Autodesk Inventor part; units mm, degrees
ref_plane "YZ Plane" through (0, 0, 0) normal (1, 0, 0) x (0, 1, 0)
ref_plane "XZ Plane" through (0, 0, 0) normal (0, 1, 0) x (-1, 0, 0)
ref_plane "XY Plane" through (0, 0, 0) normal (0, 0, 1) x (1, 0, 0)
sketch "Sketch9" plane through (0, 0, 0) normal (0, 1, 0) x (-1, 0, 0)
  line L0 (25, 25) -> (-25, 25)
  line L1 (-25, 25) -> (-25, -25)
  line L2 (-25, -25) -> (25, -25)
  line L3 (25, -25) -> (25, 25)
  line L4 (25, 25) -> (-25, -25) construction
  line L5 (-25, 25) -> (25, -25) construction
  line L6 (-23, 23) -> (23, 23)
  line L7 (23, 23) -> (23, -23)
  line L8 (23, -23) -> (-23, -23)
  line L9 (-23, -23) -> (-23, 23)
  point P0 (0, 0)
  dimension "d172" = 50
  dimension "d173" = 50
  dimension "d174" = 2
extrude "Extrusion3" add sketch "Sketch9" against normal blind 1180
sketch "Sketch10" plane through (0, 0, 0) normal (1, 0, 0) x (0, 1, 0)
  line L0 (0, 25) -> (0, -25) construction
  line L1 (0, 25) -> (-1180, 25) construction
  line L2 (-1180, -25) -> (-1180, 25) construction
  line L3 (0, -25) -> (-1180, -25) construction
  line L4 (-1175, 8.5) -> (-1158, 8.5)
  line L5 (-1158, 8.5) -> (-1158, -8.5)
  line L6 (-1158, -8.5) -> (-1175, -8.5)
  line L7 (-1175, -8.5) -> (-1175, 8.5)
  line L8 (-1175, 8.5) -> (-1158, -8.5) construction
  line L9 (-1158, 8.5) -> (-1175, -8.5) construction
  circle A0 centre (-1166.5, 0) radius 8.5
  line L10 (0, 25) -> (0, -25)
  point P0 (0, 0)
  point P1 (0, 0)
  point P2 (-1180, 0)
  dimension "d177" = 17
  dimension "d178" = 17
  dimension "d191" = 5
extrude "Extrusion4" cut sketch "Sketch10" along normal through all contours A0
pattern_linear "Rectangular Pattern4" count 10 spacing 125 along (0, 1, 0) of "Extrusion4"
properties part number "TKS 3533 FDS WAY tube3" material "Stainless Steel"
Part model, mm, in its own coordinate system. A direction names the side the tool comes from. Coordinates: 2 decimals unless noted, no trailing zeros. Order: outer loops, then holes, each group sorted by start corner. A loop starts at its lowest first (then second) coordinate and runs counter-clockwise, first axis right, second up. Notation, with made-up numbers: (-26, 42.25) - (-17, 42.25) arc R27 cw to (-17, 72.25) - close; hole circle Ø3 at (-13, 10.25). An arc over 180 degrees is marked (long way). Return JSON: item names as keys, results as strings. Group by question number.
Item 1: Cut at B-B (y = -941). List the corners of the cut face in (x, z).
Item 2: Which spindle directions (+Z, -Z, +X, -X, +Y, -Y) get a long thin tool onto all of the face, cutting with end or side? Do faces 4 (the face through (-23, -582, 0)), 5 (the face through (-25, -582, 0)). Say none if no direction does.
Item 3: Cut at C-C (z = 0). State how many separate pieces and enclosed holes the cut face has, plus the area to 3 significant figures.
Item 4: Pin check, flat tip, straight feed: pin 1 (10 mm diameter, centred on y = -416.5, z = 0, fed in from +X). Stop position of the tip, or through.
Item 5: Pull direction X, two halves, no side cores. Call faces 1 (the face through (25, -582, 0)), 2 (the face through (2, 0, -24)), 3 (the face through (23, -582, 0)): pulls with the +X half, pulls with the -X half, needs draft (parallel to the pull), parting line crosses it, or undercut.
Item 6: Drill centre lines: probe 1 along Z at (x, y) = (-17, -574.5); probe 2 along Z at (x, y) = (24, -916). Where is each one in solid material? Low to high. Write a range as from..to.
Item 7: Cut at A-A (x = 12). List the corners of the cut face in (y, z).
Check values:
{
 "1": {"outline": "(-25, -25) - (25, -25) - (25, 25) - (-25, 25) - close; hole (-23, -23) - (23, -23) - (23, 23) - (-23, 23) - close"},
 "2": {"face 4": "+Y, -Y", "face 5": "+Z, -Z, -X, +Y, -Y"},
 "3": {"separate pieces": "12", "enclosed holes": "0", "area": "4,380 mm2"},
 "4": {"pin 1": "stops at x = -23"},
 "5": {"face 1": "pulls with the +X half", "face 2": "needs draft", "face 3": "undercut"},
 "6": {"probe 1": "z = -25..-23, 23..25", "probe 2": "z = -25..-8.49, 8.49..25"},
 "7": {"outline": "(-1180, -25) - (0, -25) - (0, -23) - (-1180, -23) - close; (-1180, 23) - (0, 23) - (0, 25) - (-1180, 25) - close"}
}
